from build123d import *

# Parameters (mm, degrees)
SKETCH1_W               = 96
SKETCH1_H               = 67.5
BOSS_EXTRUDE1_DEPTH     = 1.6
CUT_EXTRUDE1_REACH      = 119.366
SKETCH2_R               = 1.5
CUT_EXTRUDE2_DEPTH      = 118.366136513
CUT_EXTRUDE2_DEPTH_BACK = 118.366136513
SKETCH3_W               = 72
SKETCH3_H               = 27


with BuildPart() as part:
    # Sketch1 → Boss-Extrude1 (new body)
    with BuildSketch(Plane(origin=(0, 0, 0), x_dir=(1, 0, 0), z_dir=(0, 1, 0))):
        with Locations((48, 33.75)):
            Rectangle(SKETCH1_W, SKETCH1_H)
    extrude(amount=BOSS_EXTRUDE1_DEPTH)

    # Sketch2 → Cut-Extrude1 (cut, up to next)
    with BuildSketch(Plane(origin=(0, 1.6, 0), x_dir=(1, 0, 0), z_dir=(0, 1, 0)), mode=Mode.PRIVATE) as cut_extrude1_sk1:
        with Locations(Location((3.96, 3.85, 0), (0, 0, 270))):
            Circle(SKETCH2_R)
    cut_extrude1_tool1 = extrude(cut_extrude1_sk1.sketch, amount=-CUT_EXTRUDE1_REACH, mode=Mode.PRIVATE) & part.part
    # Sketch2 → Cut-Extrude1 (cut, up to next)
    with BuildSketch(Plane(origin=(0, 1.6, 0), x_dir=(1, 0, 0), z_dir=(0, 1, 0)), mode=Mode.PRIVATE) as cut_extrude1_sk2:
        with Locations(Location((92.3, 3.85, 0), (0, 0, 270))):
            Circle(SKETCH2_R)
    cut_extrude1_tool2 = extrude(cut_extrude1_sk2.sketch, amount=-CUT_EXTRUDE1_REACH, mode=Mode.PRIVATE) & part.part
    # Sketch2 → Cut-Extrude1 (cut, up to next)
    with BuildSketch(Plane(origin=(0, 1.6, 0), x_dir=(1, 0, 0), z_dir=(0, 1, 0)), mode=Mode.PRIVATE) as cut_extrude1_sk3:
        with Locations(Location((3.96, 63.39, 0), (0, 0, 270))):
            Circle(SKETCH2_R)
    cut_extrude1_tool3 = extrude(cut_extrude1_sk3.sketch, amount=-CUT_EXTRUDE1_REACH, mode=Mode.PRIVATE) & part.part
    # Sketch2 → Cut-Extrude1 (cut, up to next)
    with BuildSketch(Plane(origin=(0, 1.6, 0), x_dir=(1, 0, 0), z_dir=(0, 1, 0)), mode=Mode.PRIVATE) as cut_extrude1_sk4:
        with Locations(Location((92.3, 63.39, 0), (0, 0, 270))):
            Circle(SKETCH2_R)
    cut_extrude1_tool4 = extrude(cut_extrude1_sk4.sketch, amount=-CUT_EXTRUDE1_REACH, mode=Mode.PRIVATE) & part.part
    add(cut_extrude1_tool1.solids().sort_by_distance((3.96, 1.6, -3.85))[0], mode=Mode.SUBTRACT)
    add(cut_extrude1_tool2.solids().sort_by_distance((92.3, 1.6, -3.85))[0], mode=Mode.SUBTRACT)
    add(cut_extrude1_tool3.solids().sort_by_distance((3.96, 1.6, -63.39))[0], mode=Mode.SUBTRACT)
    add(cut_extrude1_tool4.solids().sort_by_distance((92.3, 1.6, -63.39))[0], mode=Mode.SUBTRACT)

    # Sketch3 → Cut-Extrude2 (cut, two sides: drawn at the far end of the back side and taken through both)
    with BuildSketch(Plane(origin=(0, 1.6, 0), x_dir=(1, 0, 0), z_dir=(0, 1, 0)).offset(-CUT_EXTRUDE2_DEPTH_BACK)):
        with Locations((48, 41)):
            Rectangle(SKETCH3_W, SKETCH3_H)
    extrude(amount=CUT_EXTRUDE2_DEPTH + CUT_EXTRUDE2_DEPTH_BACK, mode=Mode.SUBTRACT)


solid = part.part
For this review, take the finished solid that the model builds, in its own axes (mm). Coordinates: 2 decimals unless noted, no trailing zeros. Loops run counter-clockwise (first coordinate to the right, second up) from the corner with the lowest first, then second, coordinate; pieces in that order, holes last. Notation, with made-up numbers: (88, 86.25) - (125, 86.25) arc R18 cw to (125, 97.25) - close; hole circle Ø7 at (-16.75, 74). An arc over 180 degrees is marked (long way). Use a Markdown table: item, result. Add a question column.
Item 1: We need section B-B (y = 0.95). Give the boundary of the cut face in (x, z).
Item 2: We need section C-C (z = -63.39). Give the boundary of the cut face in (x, y), and give its area (3 significant figures).
Item 3: For line 1 (X direction, y = 0.75, z = -3.85); line 2 (Z direction, x = 92.3, y = 0.45); line 3 (X direction, y = 0.8, z = -51.5), list the stretches that pass through material, from the lowest coordinate up.
Item 4: We need section D-D (x = 40). Give the boundary of the cut face in (y, z), and give its area (3 significant figures).
Item 5: Mouldability with a two-part tool opening along Z and no side actions: class faces 1 (the face through (90.97, 0.81, -3.16)), 2 (the face through (47, 1.6, -27)), 3 (the face through (4.03, 0.81, -64.89)) as pulls with the +Z half, pulls with the -Z half, needs draft (parallel to the pull), parting line crosses it, or undercut.
Item 6: We need section A-A (x = 3.96). Give the boundary of the cut face in (y, z), and give its area (3 significant figures).
Results list:
| question | item | result |
|---|---|---|
| 1 | outline | (0, -67.5) - (96, -67.5) - (96, 0) - (0, 0) - close; hole circle Ø3 at (3.96, -63.39); hole circle Ø3 at (3.96, -3.85); hole (12, -54.5) - (84, -54.5) - (84, -27.5) - (12, -27.5) - close; hole circle Ø3 at (92.3, -63.39); hole circle Ø3 at (92.3, -3.85) |
| 2 | outline | (0, 0) - (2.46, 0) - (2.46, 1.6) - (0, 1.6) - close; (5.46, 0) - (90.8, 0) - (90.8, 1.6) - (5.46, 1.6) - close; (93.8, 0) - (96, 0) - (96, 1.6) - (93.8, 1.6) - close |
| 2 | area | 144 mm^2 |
| 3 | line 1 | x = 0 to 2.46, 5.46 to 90.8, 93.8 to 96 |
| 3 | line 2 | z = -67.5 to -64.89, -61.89 to -5.35, -2.35 to 0 |
| 3 | line 3 | x = 0 to 12, 84 to 96 |
| 4 | outline | (0, -67.5) - (1.6, -67.5) - (1.6, -54.5) - (0, -54.5) - close; (0, -27.5) - (1.6, -27.5) - (1.6, 0) - (0, 0) - close |
| 4 | area | 64.8 mm^2 |
| 5 | face 1 | undercut |
| 5 | face 2 | needs draft |
| 5 | face 3 | undercut |
| 6 | outline | (0, -67.5) - (1.6, -67.5) - (1.6, -64.89) - (0, -64.89) - close; (0, -61.89) - (1.6, -61.89) - (1.6, -5.35) - (0, -5.35) - close; (0, -2.35) - (1.6, -2.35) - (1.6, 0) - (0, 0) - close |
| 6 | area | 98.4 mm^2 |
